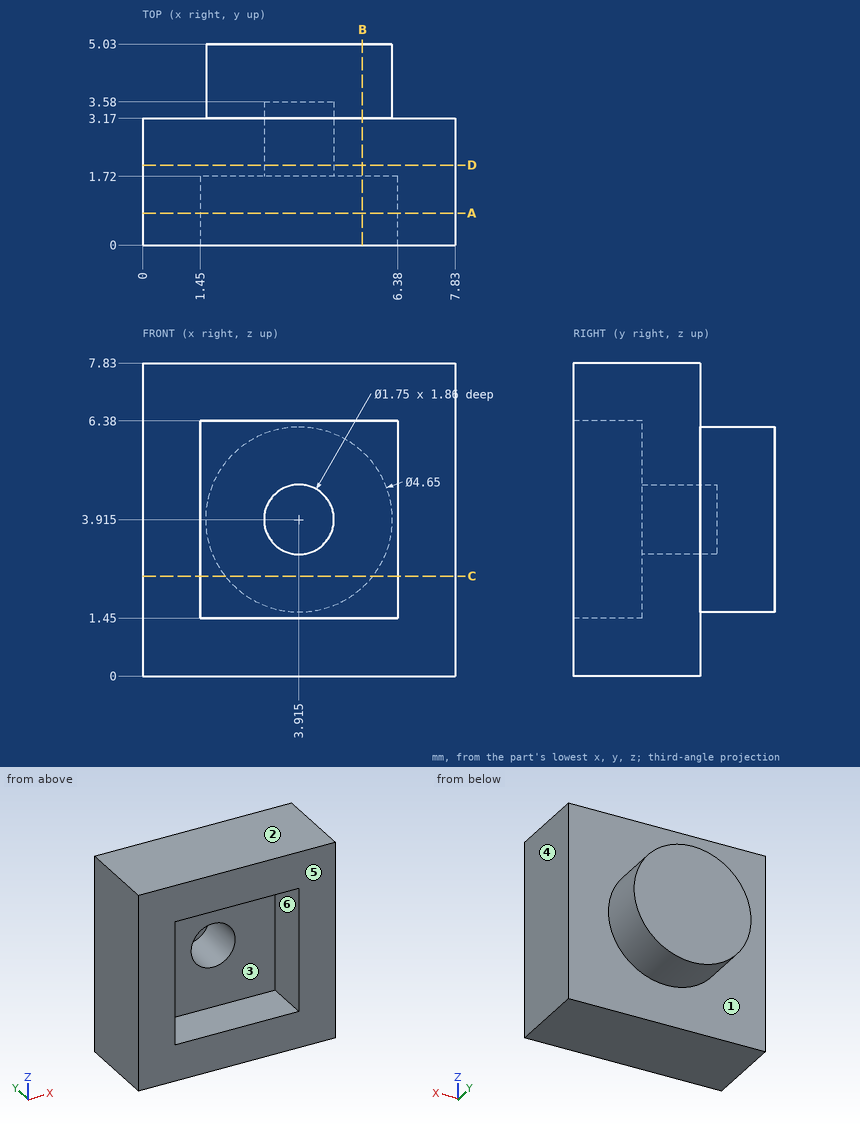
Design review of the part shown in the three views and the two pictorial views. Dimensions are in mm from the part's minimum x, y and z. A direction names the side the tool comes from. Round coordinates to 2 decimals unless told otherwise and drop trailing zeros. Write each loop counter-clockwise with the first axis right and the second up, starting at its lowest first coordinate (ties: lowest second). Pieces come first, ordered by that corner, then holes. Notation, with made-up numbers: (-3.75, 24) - (2.25, 24) arc R13 ccw to (2.25, 33) - close; hole circle Ø8 at (73, 49.25). An arc over 180 degrees is marked (long way). Answer as CSV lines item,"result". Start each with the question number.
(1) Add section A-A, the plane y = 0.8. State the section outline as (x, z) points.
(2) Add section C-C, the plane z = 2.5. State the section outline as (x, y) points, plus the area to 3 significant figures.
(3) Add section D-D, the plane y = 2. State the section outline as (x, z) points (3 decimals).
(4) For line 1 (Z direction, x = 5, y = 1.65); line 2 (Y direction, x = 4, z = 4.75), list the stretches that pass through material, from the lowest coordinate up.
(5) For pin 1 (1.4 mm diameter, centred on x = 4.5, y = 0.5, fed in from -Z); pin 2 (0.9 mm diameter, centred on x = 4, z = 4, fed in from -Y); pin 3 (2 mm diameter, centred on x = 3.915, z = 3.915, fed in from -Y), all flat-tipped, find the tip position at first contact; note any pin that passes through.
(6) Add section B-B, the plane x = 5.5. State the section outline as (y, z) points.
(7) Machinability: for the marked faces 1, 2 and 3, which of the approach directions +Z, -Z, +X, -X, +Y, -Y give a long, thin tool a straight path to every point of the face, cutting with its end or side? Answer none if there is none.
(8) Mouldability with a two-part tool opening along X and no side actions: class the marked faces 4, 5 and 6 as +X half, -X half, draft (parallel to the pull), parting line (faces both ways), or undercut.
From the geometry:
1,outline,"(0, 0) - (7.83, 0) - (7.83, 7.83) - (0, 7.83) - close; hole (1.45, 1.45) - (6.38, 1.45) - (6.38, 6.38) - (1.45, 6.38) - close"
2,outline,"(0, 0) - (1.45, 0) - (1.45, 1.72) - (6.38, 1.72) - (6.38, 0) - (7.83, 0) - (7.83, 3.17) - (5.76, 3.17) - (5.76, 5.03) - (2.07, 5.03) - (2.07, 3.17) - (0, 3.17) - close"
2,area,"23.2 mm²"
3,outline,"(0, 0) - (7.83, 0) - (7.83, 7.83) - (0, 7.83) - close; hole circle Ø1.75 at (3.915, 3.915)"
4,line 1,"z = 0 to 1.45, 6.38 to 7.83"
4,line 2,"y = 3.58 to 5.03"
5,pin 1,"stops at z = 0"
5,pin 2,"stops at y = 3.58"
5,pin 3,"stops at y = 1.72"
6,outline,"(0, 0) - (3.17, 0) - (3.17, 2.21) - (5.03, 2.21) - (5.03, 5.62) - (3.17, 5.62) - (3.17, 7.83) - (0, 7.83) - (0, 6.38) - (1.72, 6.38) - (1.72, 1.45) - (0, 1.45) - close"
7,face 1,"+Y"
7,face 2,"+Z, +X, -X, +Y, -Y"
7,face 3,"-Y"
8,face 4,"+X half"
8,face 5,"draft"
8,face 6,"undercut"
